```python
from build123d import *

# Parameters (mm, degrees)
SKETCH1_R           = 1.55
BOSS_EXTRUDE1_DEPTH = 2


with BuildPart() as part:
    # Sketch1 → Boss-Extrude1 (new body)
    with BuildSketch(Plane(origin=(0, 0, 0), x_dir=(1, 0, 0), z_dir=(0, 1, 0))):
        with BuildLine():
            ThreePointArc((-23.146596832, -42.890430613), (-19.535637384, -48.028209829), (-13.573435866, -50))
            Line((-13.573435866, -50), (13.573435866, -50))
            ThreePointArc((13.573435866, -50), (19.535637384, -48.028209829), (23.146596832, -42.890430613))
            Line((23.146596832, -42.890430613), (30.39694829, -18.877129184))
            ThreePointArc((30.39694829, -18.877129184), (30.508221739, -17.693159259), (30.150742695, -16.558974398))
            Line((30.150742695, -16.558974398), (23.672863187, -4.836752006))
            ThreePointArc((23.672863187, -4.836752006), (22.425338839, 0), (23.672863187, 4.836752006))
            Line((23.672863187, 4.836752006), (30.150742695, 16.558974398))
            ThreePointArc((30.150742695, 16.558974398), (30.508221739, 17.693159259), (30.39694829, 18.877129184))
            Line((30.39694829, 18.877129184), (23.146596832, 42.890430613))
            ThreePointArc((23.146596832, 42.890430613), (19.535637384, 48.028209829), (13.573435866, 50))
            Line((13.573435866, 50), (-13.573435866, 50))
            ThreePointArc((-13.573435866, 50), (-19.535637384, 48.028209829), (-23.146596832, 42.890430613))
            Line((-23.146596832, 42.890430613), (-30.39694829, 18.877129184))
            ThreePointArc((-30.39694829, 18.877129184), (-30.508221739, 17.693159259), (-30.150742695, 16.558974398))
            Line((-30.150742695, 16.558974398), (-23.672863187, 4.836752006))
            ThreePointArc((-23.672863187, 4.836752006), (-22.425338839, 0), (-23.672863187, -4.836752006))
            Line((-23.672863187, -4.836752006), (-30.150742695, -16.558974398))
            ThreePointArc((-30.150742695, -16.558974398), (-30.508221739, -17.693159259), (-30.39694829, -18.877129184))
            Line((-30.39694829, -18.877129184), (-23.146596832, -42.890430613))
        make_face()
        with BuildLine():
            ThreePointArc((10, -34.438564592), (0, -44.438564592), (-10, -34.438564592))
            Line((-10, -34.438564592), (-10, -11.180339887))
            ThreePointArc((-10, -11.180339887), (-15, 0), (-10, 11.180339887))
            Line((-10, 11.180339887), (-10, 34.438564592))
            ThreePointArc((-10, 34.438564592), (0, 44.438564592), (10, 34.438564592))
            Line((10, 34.438564592), (10, 11.180339887))
            ThreePointArc((10, 11.180339887), (15, 0), (10, -11.180339887))
            Line((10, -11.180339887), (10, -34.438564592))
        make_face(mode=Mode.SUBTRACT)
        with Locations(Location((-27.525, -18.01, 0), (0, 0, 270))):
            Circle(SKETCH1_R, mode=Mode.SUBTRACT)
        with Locations(Location((27.525, -18.01, 0), (0, 0, 270))):
            Circle(SKETCH1_R, mode=Mode.SUBTRACT)
        with Locations(Location((-27.525, 18.01, 0), (0, 0, 270))):
            Circle(SKETCH1_R, mode=Mode.SUBTRACT)
        with Locations(Location((27.525, 18.01, 0), (0, 0, 270))):
            Circle(SKETCH1_R, mode=Mode.SUBTRACT)
    extrude(amount=BOSS_EXTRUDE1_DEPTH)


solid = part.part
```
Check sheet for the modelled part. Datum: model origin and axes. Units: mm. A direction names the side the tool comes from. Coordinates: 2 decimals unless noted, no trailing zeros. Write each loop counter-clockwise with the first axis right and the second up, starting at its lowest first coordinate (ties: lowest second). Pieces come first, ordered by that corner, then holes. Notation, with made-up numbers: M 56,26 L 101,26 A21 cw 101,63 Z; hole C 63.25,78 d2. An arc over 180 degrees is marked long. Use one line per item in the form item = value.
Item 1: Sectioned sample at B-B, the plane z = 23. Record the cut outline in (x, y).
Answer below:
outline = M -29.15,0 L -10,0 L -10,2 L -29.15,2 Z; M 10,0 L 29.15,0 L 29.15,2 L 10,2 Z
Item 2: Sectioned sample at A-A, the plane x = 0. Record the cut outline in (y, z), and give its area (3 significant figures).
Answer below:
outline = M 0,-50 L 2,-50 L 2,-44.44 L 0,-44.44 Z; M 0,44.44 L 2,44.44 L 2,50 L 0,50 Z
area = 22.2 mm^2
Item 3: Material ranges on L1, parallel to X at y = 0.5, z = 18.01 (3 decimals); L2, parallel to X at y = 1.05, z = 18.5; L3, parallel to Z at x = -3.5, y = 0.6, recorded low to high. Write a range as from..to.
Answer below:
L1 = -30.525..-29.075, -25.975..-10, 10..25.975, 29.075..30.525
L2 = -30.48..-29, -26.05..-10, 10..26.05, 29..30.48
L3 = -50..-43.81, 43.81..50
Item 4: Set-up check for faces 4 (the face through (19.464, 0.986, 48.081)), 5 (the face through (13, 2, -12)), 6 (the face through (-26.957, 0.986, -10.78)), 7 (the face through (26.957, 0.986, 10.78)), 8 (the face through (-0.22, 0.986, -44.436)): record each of +Z, -Z, +X, -X, +Y, -Y from which the full face is reachable in a straight line by a thin tool's end or side.
Answer below:
face_4 = +Z, +X, +Y, -Y
face_5 = +Z, -Z, +X, -X, +Y
face_6 = -X, +Y, -Y
face_7 = +X, +Y, -Y
face_8 = +Y, -Y
Item 5: Gauge pin test, flat end, axial feed: pin 1 Ø1 at (y, z) = (1, -22) entering from +X (3 decimals). Record the tip position at first contact, or that the pin passes through.
Answer below:
pin_1 = 29.605
Item 6: Release check for a two-part mould opening along Z. For faces 1 (the face through (19.61, 0.99, -47.97)), 2 (the face through (0.22, 0.986, 44.436)), 3 (the face through (-26.82, 0.99, 30.72)) record: pulls with the +Z half, pulls with the -Z half, needs draft (parallel to the pull), parting line crosses it, or undercut.
Answer below:
face_1 = pulls with the -Z half
face_2 = undercut
face_3 = pulls with the +Z half
Item 7: Sectioned sample at C-C, the plane y = 1.5. State how many separate pieces and enclosed holes the cut face has, and give its area (3 significant figures).
Answer below:
separate_pieces = 1
enclosed_holes = 5
area = 3,270 mm^2
Item 8: Sectioned sample at D-D, the plane x = 17.5. Record the cut outline in (y, z), and give its area (3 significant figures).
Answer below:
outline = M 0,-49.2 L 2,-49.2 L 2,49.2 L 0,49.2 Z
area = 197 mm^2
